```python
from build123d import *

# Parameters (mm, degrees)
BOSS_EXTRUDE1_DEPTH = 5
SKETCH4_R           = 30
CUT_EXTRUDE1_DEPTH  = 115.455231423


with BuildPart() as part:
    # Sketch1 → Revolve1 (revolve)
    with BuildSketch(Plane.XY, mode=Mode.PRIVATE) as revolve1_sk:
        with BuildLine():
            Line((0, 45), (-50, 45))
            Line((-50, 45), (-50, 40))
            Line((-50, 40), (-35, 40))
            Line((-35, 40), (-35, 35))
            Line((-35, 35), (-33.5, 35))
            Line((-33.5, 35), (-33.5, 24.584524053))
            Line((-33.5, 24.584524053), (-45.163739899, 5.144957554))
            ThreePointArc((-45.163739899, 5.144957554), (-46.588810642, 0), (-45.163739899, -5.144957554))
            Line((-45.163739899, -5.144957554), (-33.5, -24.584524053))
            Line((-33.5, -24.584524053), (-33.5, -35))
            Line((-33.5, -35), (-35, -35))
            Line((-35, -35), (-35, -40))
            Line((-35, -40), (-50, -40))
            Line((-50, -40), (-50, -45))
            Line((-50, -45), (0, -45))
            Line((0, -45), (0, 45))
        make_face()
    revolve(revolve1_sk.sketch.rotate(Axis((0, 78.93258427, 0), (0, -1, 0)), 270), axis=Axis((0, 78.93258427, 0), (0, -1, 0)))

    # Sketch2 → Boss-Extrude1 (add)
    with BuildSketch(Plane(origin=(0, 35, 0), x_dir=(1, 0, 0), z_dir=(0, 1, 0))):
        with BuildLine():
            Line((-5, 36.66060556), (-5, 34.641016151))
            ThreePointArc((-5, 34.641016151), (0, 35), (5, 34.641016151))
            Line((5, 34.641016151), (5, 36.66060556))
            ThreePointArc((5, 36.66060556), (0, 37), (-5, 36.66060556))
        make_face()
    extrude(amount=BOSS_EXTRUDE1_DEPTH)

    # Sketch4 → Cut-Extrude1 (cut, through all)
    with BuildSketch(Plane.XZ.offset(45)):
        with Locations(Location((0, 0, 0), (0, 0, 270))):
            Circle(SKETCH4_R)
    extrude(amount=-CUT_EXTRUDE1_DEPTH, mode=Mode.SUBTRACT)


solid = part.part
```
Model file for the job. Use its own axes, mm. A direction names the side the tool comes from. Coordinates: 2 decimals unless noted, no trailing zeros. Write each loop counter-clockwise with the first axis right and the second up, starting at its lowest first coordinate (ties: lowest second). Pieces come first, ordered by that corner, then holes. Notation, with made-up numbers: (71.5, -30) - (122.5, -30) arc R31 cw to (122.5, -1) - close; hole circle Ø11 at (35.25, -8.5). An arc over 180 degrees is marked (long way). One line per question, with ' | ' between items. Start each with the question number.
Q1. Cut at C-C, the plane y = 8. List the corners of the cut face in (x, z), then the cut area to 3 significant figures.
Q2. Cut at B-B, the plane y = 18. List the corners of the cut face in (x, z).
Q3. 3-axis set-ups, long thin cutter, end or side, ignore diameter. For faces 4 (the face through (34, -35, 0)), 5 (the face through (-15.02, 42.46, 47.69)), 6 (the face through (0, 37, -37)): which of +Z, -Z, +X, -X, +Y, -Y reach the whole face in a straight line?
Q4. Drill centre lines: line 1 (Y direction, x = -30, z = -36.5); line 2 (Y direction, x = 6, z = 42.5); line 3 (Y direction, x = 34, z = 7). Where is each one in solid material? Low to high. Write a range as [from, to].
Q5. Pull direction Y, two halves, no side cores. Call faces 1 (the face through (22, 45, -22)), 2 (the face through (22, -45, 22)), 3 (the face through (29.7, 29.7, 15.5)): pulls with the +Y half, pulls with the -Y half, needs draft (parallel to the pull), parting line crosses it, or undercut.
Q6. Pin check, flat tips, straight feed: pin 1 (6 mm diameter, centred on x = 8.5, y = 24, fed in from +Z); pin 2 (6 mm diameter, centred on y = -10, z = 26.5, fed in from -X); pin 3 (3 mm diameter, centred on y = 20, z = 14, fed in from +X). Stop position of each tip, or through.
Answer below:
1) outline: circle Ø86.9 at (0, 0); hole circle Ø60 at (0, 0) | area: 3,100 mm^2
2) outline: circle Ø74.9 at (0, 0); hole circle Ø60 at (0, 0)
3) face 4: none | face 5: +Y, -Y | face 6: -Z
4) line 1: [-45, -40], [40, 45] | line 2: [-45, -40], [-8.88, 8.88], [40, 45] | line 3: [-45, -35], [-22.56, 22.56], [35, 45]
5) face 1: pulls with the +Y half | face 2: pulls with the -Y half | face 3: undercut
6) pin 1: z = 34.75 | pin 2: x = -36.06 | pin 3: x = 34.58
